```python
from build123d import *

# Parameters (mm, degrees)
BOX014_W     = 111
BOX014_H     = 170
BOX014_DEPTH = 1
BOX015_W     = 14
BOX015_H     = 31
BOX015_DEPTH = 1
BOX016_W     = 7
BOX016_H     = 12
BOX016_DEPTH = 1
BOX017_W     = 97
BOX017_H     = 163
BOX017_DEPTH = 1


with BuildPart() as part:
    # Box014 → Box014 (join)
    with BuildSketch(Plane.XY):
        with Locations((55.5, 85)):
            Rectangle(BOX014_W, BOX014_H)
    extrude(amount=BOX014_DEPTH)

    # Box015 → Box015 (join)
    with BuildSketch(Plane(origin=(111, 66, 0), x_dir=(1, 0, 0), z_dir=(0, 0, 1))):
        with Locations((7, 15.5)):
            Rectangle(BOX015_W, BOX015_H)
    extrude(amount=BOX015_DEPTH)

    # Box016 → Box016 (join)
    with BuildSketch(Plane(origin=(125, 77, 0), x_dir=(1, 0, 0), z_dir=(0, 0, 1))):
        with Locations((3.5, 6)):
            Rectangle(BOX016_W, BOX016_H)
    extrude(amount=BOX016_DEPTH)

    # Box017 → Box017 (join)
    with BuildSketch(Plane(origin=(3, 3, 0), x_dir=(1, 0, 0), z_dir=(0, 0, 1))):
        with Locations((48.5, 81.5)):
            Rectangle(BOX017_W, BOX017_H)
    extrude(amount=BOX017_DEPTH)


with BuildPart() as part_1:
    # Body002 placement: moved
    add(part.part.moved(Location((24, 3, 6))))


solid = part_1.part
```
For this review, take the finished solid that the model builds, in its own axes (mm). Coordinates: 2 decimals unless noted, no trailing zeros. Loops run counter-clockwise (first coordinate to the right, second up) from the corner with the lowest first, then second, coordinate; pieces in that order, holes last.
1. Insertion check: P1, Ø0.5, axis at x = 154, z = 6.5, coming from the -Y side; P2, Ø0.5, axis at y = 97.5, z = 6.5, coming from the +X side; P3, Ø0.5, axis at y = 119.5, z = 6.5, coming from the +X side. Each pin has a flat end and moves straight along its axis. Give the tip position at first contact, or say it passes through.
2. For line 1 (X direction, y = 109, z = 6.3); line 2 (Y direction, x = 140, z = 6.25), list the stretches that pass through material, from the lowest coordinate up.
3. Add section B-B, the plane y = 107. Give the boundary of the cut face in (x, z).
4. Add section A-A, the plane z = 6.45. Give the boundary of the cut face in (x, y), then the cut area to 3 significant figures.
Result:
1. P1: stops at y = 80
1. P2: stops at x = 149
1. P3: stops at x = 135
2. line 1: x = 24 to 135
2. line 2: y = 69 to 100
3. outline: (24, 6) - (135, 6) - (135, 7) - (24, 7) - close
4. outline: (24, 3) - (135, 3) - (135, 69) - (149, 69) - (149, 80) - (156, 80) - (156, 92) - (149, 92) - (149, 100) - (135, 100) - (135, 173) - (24, 173) - close
4. area: 19,400 mm2
